```python
from build123d import *

# Parameters (mm, degrees)
F1_DEPTH = 30
F2_R     = 4
F3_DEPTH = 30.001
F4_SIZE  = 0.5
F5_R     = 4.25
F6_DEPTH = 146.001


with BuildPart() as f1:
    # F0 (on Right) → F1 (new body)
    with BuildSketch(Plane.YZ):
        Polygon((10, 0), (10, 136), (192, 136), (192, 146), (0, 146), (-20, 146), (-20, 136), (0, 136), (0, 0), align=None)
    extrude(amount=F1_DEPTH)

    # F2 (on face) → F3 (cut, through all)
    with BuildSketch(Plane(origin=(0, 10, 0), x_dir=(-1, 0, 0), z_dir=(0, 1, 0))):
        with Locations((-15, 70)):
            Circle(F2_R)
        with Locations((-15, 10)):
            Circle(F2_R)
    extrude(amount=-F3_DEPTH, mode=Mode.SUBTRACT)

    # F4
    f4_edges = [f1.edges().sort_by_distance(p)[0] for p in [
        (19, 10, 70),
        (11, 5, 70),
        (19, 0, 70),
        (19, 10, 10),
        (11, 5, 10),
        (19, 0, 10),
    ]]
    chamfer(f4_edges, length=F4_SIZE)

    # F5 (on face) → F6 (cut, through all)
    with BuildSketch(Plane.XY.offset(146)):
        with Locations((15, 182)):
            Circle(F5_R)
        with Locations((15, 162)):
            Circle(F5_R)
        with Locations((15, -10)):
            Circle(F5_R)
        with Locations((15, 30)):
            Circle(F5_R)
        with Locations((15, 50)):
            Circle(F5_R)
    extrude(amount=-F6_DEPTH, mode=Mode.SUBTRACT)


solid = f1.part
```
Read the model definition and answer for the solid it produces. Units are mm, in the model's axes. A direction names the side the tool comes from. Round coordinates to 2 decimals unless told otherwise and drop trailing zeros. Write each loop counter-clockwise with the first axis right and the second up, starting at its lowest first coordinate (ties: lowest second). Pieces come first, ordered by that corner, then holes. Notation, with made-up numbers: M 13.25,-20.5 L 45.25,-20.5 A11 cw 45.25,-10.5 Z; hole C 67.5,-28 d5. An arc over 180 degrees is marked long. One line per item, written item: value.
Q1. Flat-ended cylindrical pins translate along their axes: pin 1 Ø5 at (x, y) = (15, 30) entering from +Z; pin 2 Ø10.5 at (x, z) = (15, 10) entering from +Y; pin 3 Ø3 at (x, z) = (20.5, 59) entering from -Y; pin 4 Ø2 at (x, y) = (4.5, 126) entering from -Z. Find the tip coordinate at first contact, or state that the pin passes through.
Data:
pin 1: through
pin 2: y = 10
pin 3: y = 0
pin 4: z = 136
Q2. Find section C-C on x = 7.25. Write down the section's boundary in (y, z), plus the area to 3 significant figures.
Data:
outline: M -20,136 L 0,136 L 0,0 L 10,0 L 10,136 L 192,136 L 192,146 L -20,146 Z
area: 3,480 mm2
Q3. Straight lines are drawn through the part: line 1 (Z direction, x = 15, y = 5.5); line 2 (Y direction, x = 15, z = 139.5); line 3 (Y direction, x = 18.5, z = 90.5). For each, find the intervals that lie inside material, in ascending order. Write a range as [from, to].
Data:
line 1: [0, 6], [14, 66], [74, 146]
line 2: [-20, -14.25], [-5.75, 25.75], [34.25, 45.75], [54.25, 157.75], [166.25, 177.75], [186.25, 192]
line 3: [0, 10]
Q4. For a pull along Z with two mould halves and no side action, classify faces 1 (the flat face through (15, 87, 146)), 2 (the cylindrical face through (15.867, 5.063, 66.095)), 3 (the cylindrical face through (14.08, -14.15, 141.07)), 4 (the cylindrical face through (19, 5, 10)) as +Z half, -Z half, draft (parallel to the pull), parting line (faces both ways), or undercut.
Data:
face 1: +Z half
face 2: undercut
face 3: draft
face 4: undercut
Q5. Find section B-B on z = 10. Write down the section's boundary in (x, y), plus the area to 4 significant figures.
Data:
outline: M 0,0 L 10.5,0 L 11,0.5 L 11,9.5 L 10.5,10 L 0,10 Z; M 19,0.5 L 19.5,0 L 30,0 L 30,10 L 19.5,10 L 19,9.5 Z
area: 219.5 mm2
Q6. Which of the six approach directions +Z, -Z, +X, -X, +Y, -Y give full straight-line access (tool end or side, diameter ignored) to faces 5 (the flat face through (15, 100, 136)), 6 (the flat face through (21, 0, 69)), 7 (the cylindrical face through (14.447, 186.214, 141.07))?
Data:
face 5: -Z, +X, -X, +Y
face 6: -Z, +X, -X, -Y
face 7: +Z, -Z
Q7. Find section D-D on z = 105. Write down the section's boundary in (x, y), plus the area to 3 significant figures.
Data:
outline: M 0,0 L 30,0 L 30,10 L 0,10 Z
area: 300 mm2
Q8. Find section A-A on y = 50. Write down the section's boundary in (x, z).
Data:
outline: M 0,136 L 10.75,136 L 10.75,146 L 0,146 Z; M 19.25,136 L 30,136 L 30,146 L 19.25,146 Z
